Build history of the part. All positions in model axes, mm. Face numbers are marked on the shaded views. A direction names the side the tool comes from. Give positions to 0.01 mm unless a question says otherwise; leave off trailing zeros. Loops run counter-clockwise (first coordinate to the right, second up) from the corner with the lowest first, then second, coordinate; pieces in that order, holes last. Notation, with made-up numbers: (-17.75, 36.5) -> (10.25, 36.5) arc R27 cw to (10.25, 57.5) -> close; hole circle Ø9 at (-12, 46). An arc over 180 degrees is marked (long way). Answer as a JSON object with one key per item and string values. Group by question number.
Autodesk Fusion 360 part; units mm, degrees
sketch "Sketch1" plane through (0, 0, 0) normal (0, 1, 0) x (1, 0, 0)
  line L0 (0, -25.4) -> (0, 0)
  line L1 (0, 0) -> (25.4, 0)
  line L2 (12.7, -12.7) -> (11.05, -11.05) construction
  line L3 (3.175, -25.4) -> (3.175, -3.175)
  line L4 (3.175, -3.175) -> (25.4, -3.175)
  line L5 (25.4, -3.175) -> (25.4, 0)
  line L6 (0, -25.4) -> (3.175, -25.4)
  dimension "d1" = 25.4
  dimension "d2" = 25.4
  dimension "d13" = 3.175
extrude "Extrude1" add sketch "Sketch1" along normal blind 75
hole "Hole3" at (3.175, 110.487, 14.2875) direction (-1, 0, 0) diameter 6.5 end through all
hole "Hole4" at (14.2875, 60.713, 3.175) direction (0, 0, -1) diameter 6.5 depth 30 tip angle 118
mirror "Mirror1" about plane through (0, 0, 0) normal (0, 1, 0) of bodies 1 merged
hole "Hole5" at (17.9, 0, 3.175) direction (0, 0, -1) diameter 6.5 depth 30 tip angle 118
equation "d27 = ( 22.225 / 2 ) * 1 mm"
equation "d35 = ( 22.225 / 2 ) * 1 mm"
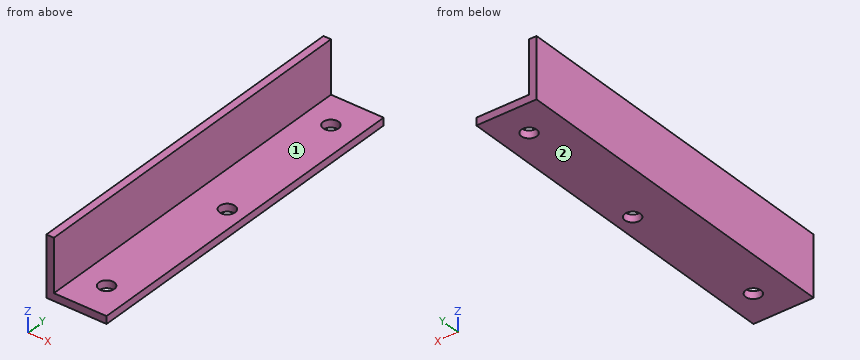
(1) Probe line 1 along Y through (x, z) = (17.9, 0.75); line 2 along X through (y, z) = (-35, 22) (3 decimals); line 3 along X through (y, z) = (0, 2.1). List the from-to ranges inside material, lowest first. Write a range as [from, to].
(2) Pin check, flat tips, straight feed: pin 1 (1 mm diameter, centred on x = 4.5, z = 22.5, fed in from +Y); pin 2 (2 mm diameter, centred on y = 55.5, z = 17, fed in from +X) (3 decimals); pin 3 (11 mm diameter, centred on x = 11, y = 19.5, fed in from +Z) (3 decimals). Stop position of each tip, or through.
(3) Saw through at B-B on y = -27. List the corners of the cut face in (x, z) (3 decimals), plus the area to 3 significant figures.
(4) 3-axis set-ups, long thin cutter, end or side, ignore diameter. For the marked faces 1 and 2: which of +Z, -Z, +X, -X, +Y, -Y reach the whole face in a straight line?
(5) Saw through at C-C on x = 7. List the corners of the cut face in (y, z) (3 decimals).
(6) Saw through at A-A on y = 0. List the corners of the cut face in (x, z) (3 decimals).
(7) Saw through at D-D on z = 18.5. List the corners of the cut face in (x, y) (3 decimals).
Calculated:
{
 "1": {"line 1": "y = [-75, -3.25], [3.25, 75]", "line 2": "x = [0, 3.175]", "line 3": "x = [0, 14.65], [21.15, 25.4]"},
 "2": {"pin 1": "passes through", "pin 2": "stops at x = 3.175", "pin 3": "stops at z = 3.175"},
 "3": {"outline": "(0, 0) -> (25.4, 0) -> (25.4, 3.175) -> (3.175, 3.175) -> (3.175, 25.4) -> (0, 25.4) -> close", "area": "151 mm^2"},
 "4": {"face 1": "+Z, +X, +Y, -Y", "face 2": "-Z, +X, -X, +Y, -Y"},
 "5": {"outline": "(-75, 0) -> (75, 0) -> (75, 3.175) -> (-75, 3.175) -> close"},
 "6": {"outline": "(0, 0) -> (14.65, 0) -> (14.65, 3.175) -> (3.175, 3.175) -> (3.175, 25.4) -> (0, 25.4) -> close; (21.15, 0) -> (25.4, 0) -> (25.4, 3.175) -> (21.15, 3.175) -> close"},
 "7": {"outline": "(0, -75) -> (3.175, -75) -> (3.175, 75) -> (0, 75) -> close"}
}
